```python
from build123d import *

# Parameters (mm, degrees)
SKETCH1_R           = 50
BOSS_EXTRUDE1_DEPTH = 15
FILLET1_R           = 10
SKETCH5_R           = 2.5
BOSS_EXTRUDE2_DEPTH = 80
FILLET2_R           = 10
SKETCH6_W           = 240
SKETCH6_H           = 150
BOSS_EXTRUDE3_DEPTH = 15
SKETCH7_W           = 195
SKETCH7_H           = 105
CUT_EXTRUDE1_DEPTH  = 15
FILLET3_R           = 10


with BuildPart() as part:
    # Sketch1 → Boss-Extrude1 (new body)
    with BuildSketch(Plane(origin=(0, 0, 0), x_dir=(1, 0, 0), z_dir=(0, 1, 0))):
        with Locations(Location((0, 0, 0), (0, 0, 270))):
            Circle(SKETCH1_R)
    extrude(amount=BOSS_EXTRUDE1_DEPTH)

    # Fillet1
    fillet1_edges = [part.edges().sort_by_distance(p)[0] for p in [
        (0, 15, -50),
    ]]
    fillet(fillet1_edges, radius=FILLET1_R)

    # Sketch3 → Cut-Revolve1 (revolve, cut)
    with BuildSketch(Plane.XY, mode=Mode.PRIVATE) as cut_revolve1_sk:
        with BuildLine():
            Line((0, 0), (40, 0))
            Line((40, 0), (40, 5))
            ThreePointArc((40, 5), (38.535533906, 8.535533906), (35, 10))
            Line((35, 10), (0, 10))
            Line((0, 10), (0, 0))
        make_face()
    revolve(cut_revolve1_sk.sketch.rotate(Axis((0, 0, 0), (0, 1, 0)), 90), axis=Axis((0, 0, 0), (0, 1, 0)), mode=Mode.SUBTRACT)

    # Sketch5 → Boss-Extrude2 (add)
    with BuildSketch(Plane(origin=(0, 15, 0), x_dir=(1, 0, 0), z_dir=(0, 1, 0))):
        with Locations(Location((0, 0, 0), (0, 0, 270))):
            Circle(SKETCH5_R)
    extrude(amount=BOSS_EXTRUDE2_DEPTH)

    # Fillet2
    fillet2_edges = [part.edges().sort_by_distance(p)[0] for p in [
        (0, 15, -2.5),
    ]]
    fillet(fillet2_edges, radius=FILLET2_R)

    # Sketch6 → Boss-Extrude3 (add, symmetric)
    with BuildSketch(Plane.XY):
        with Locations((0, 170)):
            Rectangle(SKETCH6_W, SKETCH6_H)
    extrude(amount=BOSS_EXTRUDE3_DEPTH, both=True)

    # Sketch7 → Cut-Extrude1 (cut)
    with BuildSketch(Plane.XY.offset(15)):
        with Locations((0, 170)):
            Rectangle(SKETCH7_W, SKETCH7_H)
    extrude(amount=-CUT_EXTRUDE1_DEPTH, mode=Mode.SUBTRACT)

    # Fillet3
    fillet3_edges = [part.edges().sort_by_distance(p)[0] for p in [
        (-120, 170, 15),
        (0, 95, 15),
        (120, 170, 15),
        (0, 245, 15),
    ]]
    fillet(fillet3_edges, radius=FILLET3_R)


solid = part.part
```
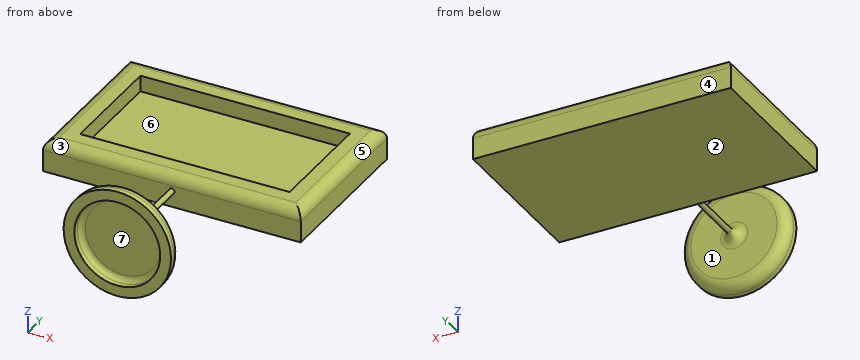
Check sheet for the modelled part. Datum: model origin and axes. Units: mm. Face numbers are marked on the shaded views. A direction names the side the tool comes from. Round coordinates to 2 decimals unless told otherwise and drop trailing zeros. Loops run counter-clockwise (first coordinate to the right, second up) from the corner with the lowest first, then second, coordinate; pieces in that order, holes last. Notation, with made-up numbers: (36, 27.5) - (54, 27.5) arc R24 cw to (54, 60.5) - close; hole circle Ø2 at (-8.5, 72). An arc over 180 degrees is marked (long way). Answer as a JSON object with one key per item and string values. Group by question number.
Q1. Sectioned sample at B-B, the plane y = 84. Enter the section's corners in (x, z).
Q2. Gauge pin test, flat ends, axial feed: P1, Ø4.5, axis at x = 47, z = 10, coming from the +Y side; P2, Ø5, axis at x = 8.5, z = -5, coming from the -Y side; P3, Ø8, axis at x = -7.5, y = 201.5, coming from the +Z side. Record the tip position at first contact, or that the pin passes through.
Q3. Mould release check, pull along X, two halves, no side actions. Record for the marked faces 4, 5, 6 and 7: released by +X, released by -X, zero draft, split by the parting line, or undercut.
Q4. Set-up check for the marked faces 1, 2 and 3: record each of +Z, -Z, +X, -X, +Y, -Y from which the full face is reachable in a straight line by a thin tool's end or side.
Q5. Scan lines: line 1 along X through (y, z) = (3, 0); line 2 along Y through (x, z) = (49, 1.5); line 3 along Y through (x, z) = (12, 29). Record each from-to range of solid material in increasing order. Write a range as [from, to].
Q6. Sectioned sample at A-A, the plane y = 177.5. Enter the section's corners in (x, z), plus the area to 3 significant figures.
Solution:
{
 "1": {"outline": "circle Ø5 at (0, 0)"},
 "2": {"P1": "stops at y = 244.61", "P2": "stops at y = 10", "P3": "stops at z = 0"},
 "3": {"face 4": "zero draft", "face 5": "released by +X", "face 6": "undercut", "face 7": "undercut"},
 "4": {"face 1": "none", "face 2": "-Z, +X, -X, +Y", "face 3": "+Z, +X, -X"},
 "5": {"line 1": "x = [-50, -40], [40, 50]", "line 2": "y = [0, 9.31], [95, 117.5], [222.5, 245]", "line 3": "y = [10, 15]"},
 "6": {"outline": "(-120, -15) - (120, -15) - (120, 5) arc R10 ccw to (110, 15) - (97.5, 15) - (97.5, 0) - (-97.5, 0) - (-97.5, 15) - (-110, 15) arc R10 ccw to (-120, 5) - close", "area": "4,230 mm²"}
}
